Input: dimensioned drawing with shaded views. Units: mm. Origin: part minimum x, y, z. A direction names the side the tool comes from. Give positions to 0.01 mm unless a question says otherwise; leave off trailing zeros. Order: outer loops, then holes, each group sorted by start corner. A loop starts at its lowest first (then second) coordinate and runs counter-clockwise, first axis right, second up.
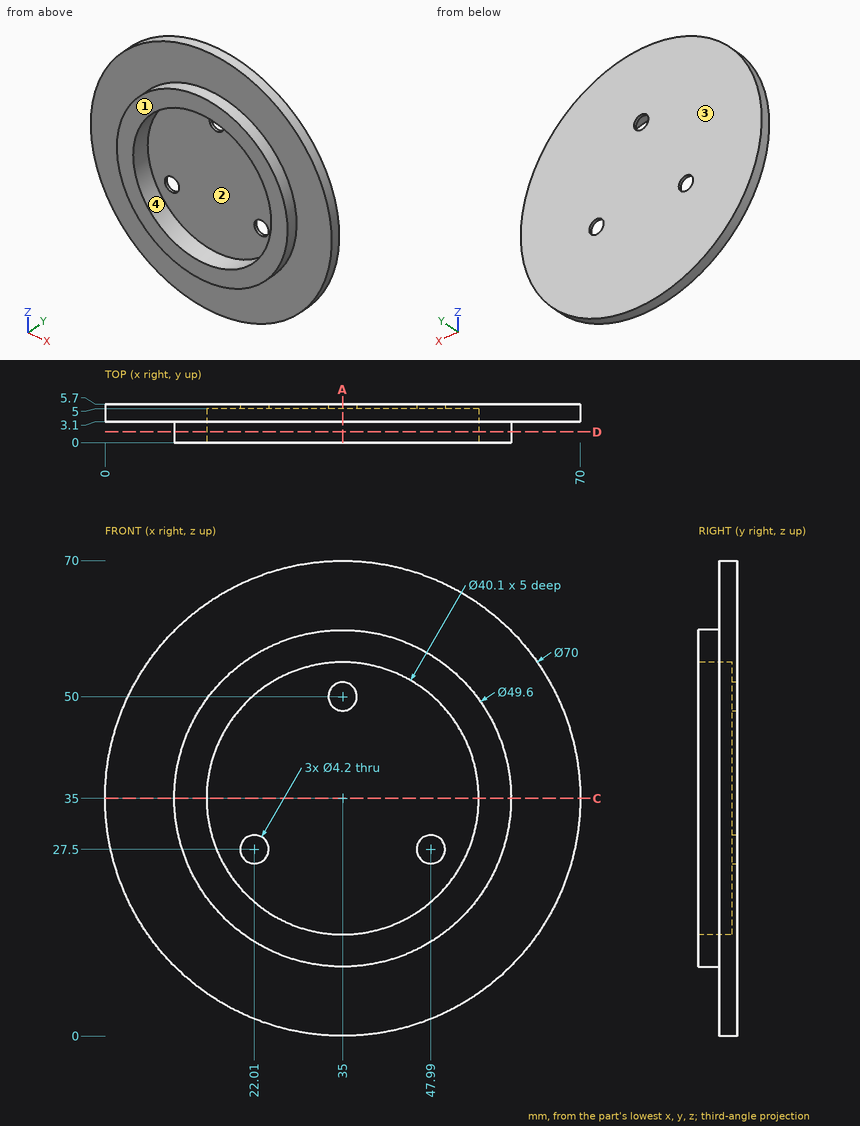
1) Section query D-D, the plane y = 1.6. Return the cut outline in (x, z), and give its area (3 significant figures).
Report:
outline: circle Ø49.6 at (35, 35); hole circle Ø40.1 at (35, 35)
area: 669 mm2
2) Pin query (flat end, axial travel): pin 1 (3 mm diameter, centred on y = 3.5, z = 53.5, fed in from +X) (1 decimal); pin 2 (12 mm diameter, centred on x = 59.5, z = 16, fed in from -Y); pin 3 (3 mm diameter, centred on x = 15, z = 40.5, fed in from -Y); pin 4 (6.5 mm diameter, centred on x = 35, z = 50, fed in from -Y). Return the tip coordinate at first contact, or that it passes through.
Report:
pin 1: stops at x = 65.6
pin 2: stops at y = 3.1
pin 3: stops at y = 0
pin 4: stops at y = 5
3) Material intervals for L1, parallel to X at y = 5.2, z = 27.5; L2, parallel to Z at x = 37.5, y = 2.8; L3, parallel to X at y = 2.65, z = 35, sorted ascending.
Report:
L1: x = 0.81 to 19.91, 24.11 to 45.89, 50.09 to 69.19
L2: z = 10.33 to 15.11, 54.89 to 59.67
L3: x = 10.2 to 14.95, 55.05 to 59.8
4) Section query A-A, the plane x = 35. Return the cut outline in (y, z).
Report:
outline: (0, 10.2) - (3.1, 10.2) - (3.1, 0) - (5.7, 0) - (5.7, 47.9) - (5, 47.9) - (5, 14.95) - (0, 14.95) - close; (0, 55.05) - (5, 55.05) - (5, 52.1) - (5.7, 52.1) - (5.7, 70) - (3.1, 70) - (3.1, 59.8) - (0, 59.8) - close
5) Reachability of the marked faces 1 and 2 from +Z, -Z, +X, -X, +Y, -Y: full face, straight path, thin tool, end or side. Return the list, or none.
Report:
face 1: +Z, -Z, +X, -X, -Y
face 2: -Y
6) Section query C-C, the plane z = 35. Return the cut outline in (x, y), and give its area (3 significant figures).
Report:
outline: (0, 3.1) - (10.2, 3.1) - (10.2, 0) - (14.95, 0) - (14.95, 5) - (55.05, 5) - (55.05, 0) - (59.8, 0) - (59.8, 3.1) - (70, 3.1) - (70, 5.7) - (0, 5.7) - close
area: 135 mm2
7) Draft query along X for the marked faces 3 and 4. Return one class per face: +X half, -X half, draft (parallel to the pull), parting line (faces both ways), or undercut.
Report:
face 3: draft
face 4: undercut
